from build123d import *

# Parameters (mm, degrees)
SKETCH_1_W      = 50
SKETCH_1_H      = 50
SKETCH_1_R      = 1.55
SKETCH_1_R_2    = 6.05
EXTRUDE_1_DEPTH = 3
FILLET_1_R      = 5


with BuildPart() as part:
    # ｽｹｯﾁ1 → ﾎﾞｽ - 押し出し1 (new body)
    with BuildSketch(Plane.XY):
        Rectangle(SKETCH_1_W, SKETCH_1_H)
        with Locations((-20, 20)):
            Circle(SKETCH_1_R, mode=Mode.SUBTRACT)
        with Locations((20, 20)):
            Circle(SKETCH_1_R, mode=Mode.SUBTRACT)
        with Locations((20, -20)):
            Circle(SKETCH_1_R, mode=Mode.SUBTRACT)
        with Locations((-20, -20)):
            Circle(SKETCH_1_R, mode=Mode.SUBTRACT)
        Circle(SKETCH_1_R_2, mode=Mode.SUBTRACT)
        with Locations((-9, 0)):
            Circle(SKETCH_1_R, mode=Mode.SUBTRACT)
        with Locations(Location((9, 0, 0), (0, 0, 180))):
            Circle(SKETCH_1_R, mode=Mode.SUBTRACT)
    extrude(amount=EXTRUDE_1_DEPTH)

    # ﾌｨﾚｯﾄ1
    fillet_1_edges = [part.edges().sort_by_distance(p)[0] for p in [
        (25, -25, 1.5),
        (-25, -25, 1.5),
        (-25, 25, 1.5),
        (25, 25, 1.5),
    ]]
    fillet(fillet_1_edges, radius=FILLET_1_R)


solid = part.part
Check sheet for the modelled part. Datum: model origin and axes. Units: mm. Give positions to 0.01 mm unless a question says otherwise; leave off trailing zeros. Loops run counter-clockwise (first coordinate to the right, second up) from the corner with the lowest first, then second, coordinate; pieces in that order, holes last. Notation, with made-up numbers: M 28.25,39.5 L 33.25,39.5 A33 ccw 33.25,74.5 Z; hole C 41,-38 d5. An arc over 180 degrees is marked long. Answer as a JSON object with one key per item and string values. Group by question number.
Q1. Go/stop test with a flat-tipped pin: P1, Ø1.9, axis at x = 20, y = -20, coming from the -Z side. Record where the tip stops, or that it passes through.
Q2. Cross-section at C-C on y = -5. Record the cut outline in (x, z).
Q3. Cross-section at A-A on x = 0. Record the cut outline in (y, z).
Q4. Release check for a two-part mould opening along Y. For faces 1 (the cylindrical face through (23, -24, 2)), 2 (the flat face through (25, 0, 1)), 3 (the cylindrical face through (20.83, -18.69, 1.48)), 4 (the cylindrical face through (23, 24, 2)) record: released by +Y, released by -Y, zero draft, split by the parting line, or undercut.
Q5. Cross-section at B-B on z = 0.6. Record the cut outline in (x, y).
Q6. Material ranges on line 1 along Y through (x, z) = (-20, 1.75); line 2 along Y through (x, z) = (3.5, 1.9); line 3 along X through (y, z) = (2, 0.9), recorded low to high. Write a range as [from, to].
Evaluation:
{
 "1": {"P1": "passes through"},
 "2": {"outline": "M -25,0 L -3.41,0 L -3.41,3 L -25,3 Z; M 3.41,0 L 25,0 L 25,3 L 3.41,3 Z"},
 "3": {"outline": "M -25,0 L -6.05,0 L -6.05,3 L -25,3 Z; M 6.05,0 L 25,0 L 25,3 L 6.05,3 Z"},
 "4": {"face 1": "released by -Y", "face 2": "zero draft", "face 3": "undercut", "face 4": "released by +Y"},
 "5": {"outline": "M -25,-20 A5 ccw -20,-25 L 20,-25 A5 ccw 25,-20 L 25,20 A5 ccw 20,25 L -20,25 A5 ccw -25,20 Z; hole C -20,-20 d3.1; hole C -20,20 d3.1; hole C -9,0 d3.1; hole C 0,0 d12.1; hole C 9,0 d3.1; hole C 20,-20 d3.1; hole C 20,20 d3.1"},
 "6": {"line 1": "y = [-25, -21.55], [-18.45, 18.45], [21.55, 25]", "line 2": "y = [-25, -4.93], [4.93, 25]", "line 3": "x = [-25, -5.71], [5.71, 25]"}
}
